from build123d import *

# Parameters (mm, degrees)
ESBO_O1_R                       = 1.75
RESSALTO_EXTRUS_O1_DEPTH        = 8
ESBO_O2_R                       = 1.65
CORTE_EXTRUS_O1_DEPTH           = 7
ESBO_O3_R                       = 1.75
CORTE_EXTRUS_O2_DEPTH           = 18.5
CORTE_EXTRUS_O3_DEPTH           = 2
CORTE_EXTRUS_O3_TAPER           = 20
CORTE_EXTRUS_O3_OTHER_WAY_DEPTH = 6


with BuildPart() as part:
    # Esboço1 → Ressalto-extrusão1 (new body)
    with BuildSketch(Plane.XY):
        with BuildLine():
            Line((17.5, 7.5), (6.986594306, 7.5))
            ThreePointArc((6.986594306, 7.5), (0, 10.25), (-6.986594306, 7.5))
            Line((-6.986594306, 7.5), (-17.5, 7.5))
            Line((-17.5, 7.5), (-17.5, -0.5))
            Line((-17.5, -0.5), (-7.232738071, -0.5))
            ThreePointArc((-7.232738071, -0.5), (-4.946589734, -5.300353762), (0, -7.25))
            Line((0, -7.25), (12.236067977, -7.25))
            Line((12.236067977, -7.25), (12.236067977, -4.75))
            Line((12.236067977, -4.75), (2.236067977, -4.75))
            ThreePointArc((2.236067977, -4.75), (-4.364690104, 2.917529829), (5.244044241, -0.25))
            Line((5.244044241, -0.25), (12.736067977, -0.25))
            Line((12.736067977, -0.25), (12.736067977, -2.25))
            Line((12.736067977, -2.25), (15.807189139, -2.25))
            Line((15.807189139, -2.25), (17.5, -2.25))
            Line((17.5, -2.25), (17.5, 7.5))
        make_face()
        with Locations((12.5, 3.5)):
            Circle(ESBO_O1_R, mode=Mode.SUBTRACT)
        with Locations((-12.5, 3.5)):
            Circle(ESBO_O1_R, mode=Mode.SUBTRACT)
    extrude(amount=RESSALTO_EXTRUS_O1_DEPTH)

    # Esboço2 → Corte-extrusão1 (cut)
    with BuildSketch(Plane(origin=(17.5, 0, 0), x_dir=(0, 0, -1), z_dir=(1, 0, 0))):
        with Locations((-4, 2.625)):
            Circle(ESBO_O2_R)
    corte_extrus_o1 = extrude(amount=-CORTE_EXTRUS_O1_DEPTH, mode=Mode.SUBTRACT)

    # Espelhar1: Corte-extrusão1 across plane
    add(corte_extrus_o1.mirror(Plane(origin=(0, 0, 0), x_dir=(0, 0, 1), z_dir=(1, 0, 0))), mode=Mode.SUBTRACT)

    # Esboço3 → Corte-extrusão2 (cut, through all)
    with BuildSketch(Plane.XZ.offset(7.25)):
        with Locations((7.85, 4)):
            Circle(ESBO_O3_R)
    extrude(amount=-CORTE_EXTRUS_O2_DEPTH, mode=Mode.SUBTRACT)

    # Esboço4 → Corte-extrusão3 (cut)
    with BuildSketch(Plane(origin=(0, 7.5, 0), x_dir=(1, 0, 0), z_dir=(0, 1, 0))):
        Polygon((11.083161507, -4), (9.466580754, -1.2), (6.233419246, -1.2), (4.616838493, -4), (6.233419246, -6.8), (9.466580754, -6.8), align=None)
    extrude(amount=-CORTE_EXTRUS_O3_DEPTH, taper=CORTE_EXTRUS_O3_TAPER, mode=Mode.SUBTRACT)

    # Esboço4 → Corte-extrusão3 other way (cut)
    with BuildSketch(Plane(origin=(0, 7.5, 0), x_dir=(1, 0, 0), z_dir=(0, 1, 0))):
        Polygon((11.083161507, -4), (9.466580754, -1.2), (6.233419246, -1.2), (4.616838493, -4), (6.233419246, -6.8), (9.466580754, -6.8), align=None)
    extrude(amount=CORTE_EXTRUS_O3_OTHER_WAY_DEPTH, mode=Mode.SUBTRACT)


solid = part.part
CAD build for the part. Positions are in the model's coordinates, mm. A direction names the side the tool comes from. Round coordinates to 2 decimals unless told otherwise and drop trailing zeros. Order: outer loops, then holes, each group sorted by start corner. A loop starts at its lowest first (then second) coordinate and runs counter-clockwise, first axis right, second up. Notation, with made-up numbers: (2.25, -4.5) -> (13.25, -4.5) arc R18 ccw to (13.25, 8.5) -> close; hole circle Ø7 at (67, 7.5). An arc over 180 degrees is marked (long way). Write item = value, one per line. Start each with the question number.
(1) Pin check, flat tips, straight feed: P1, Ø1.6, axis at y = 2, z = 3.5, coming from the -X side; P2, Ø1, axis at y = 2.5, z = 4, coming from the +X side; P3, Ø1.2, axis at y = -6.5, z = 4.5, coming from the +X side. Stop position of each tip, or through.
(2) Cut at A-A, the plane x = -12.5. List the corners of the cut face in (y, z) (3 decimals), then the cut area to 3 significant figures.
(3) Probe line 1 (Z direction, x = 7.85, y = 1.4); line 2 (X direction, y = 0.25, z = 6); line 3 (Y direction, x = 8.5, z = 7.75). List the from-to ranges inside material, lowest first. Write a range as [from, to].
(4) Pull direction Z, two halves, no side cores. Call faces 6 (the cylindrical face through (12.272, 5.235, 3.944)), 7 (the flat face through (-10.5, 3, 4)), 8 (the flat face through (0, 6, 0)), 9 (the flat face through (0, 6, 8)): released by +Z, released by -Z, zero draft, split by the parting line, or undercut.
(5) Which spindle directions (+Z, -Z, +X, -X, +Y, -Y) get a long thin tool onto all of the face, cutting with end or side? Do faces 1 (the flat face through (13, 7.5, 4)), 2 (the flat face through (6, -4.75, 3)), 3 (the flat face through (-12, 7.5, 4)), 4 (the flat face through (5.234, 8.131, 5.069)), 5 (the flat face through (10, -0.25, 4)). Say none if no direction does.
(6) Cut at B-B, the plane x = 7.85. State how many separate pieces and enclosed holes the cut face has, then the cut area to 3 significant figures.
Model answer:
q1.P1 = -10.5
q1.P2 = 10.5
q1.P3 = 12.24
q2.outline = (-0.5, 0) -> (1.75, 0) -> (1.75, 2.601) arc R1.65 cw to (1.75, 5.399) -> (1.75, 8) -> (-0.5, 8) -> close; (5.25, 0) -> (7.5, 0) -> (7.5, 8) -> (5.25, 8) -> close
q2.area = 34.5 mm2
q3.line_1 = [0, 2.25], [5.75, 8]
q3.line_2 = [-17.5, -5.24], [5.24, 17.5]
q3.line_3 = [-7.25, -4.75], [-0.25, 7.5]
q4.face_6 = zero draft
q4.face_7 = undercut
q4.face_8 = released by -Z
q4.face_9 = released by +Z
q5.face_1 = +Z, -Z, +X, +Y
q5.face_2 = +Z, -Z, +X
q5.face_3 = +Z, -Z, -X, +Y
q5.face_4 = +X, +Y
q5.face_5 = +Z, -Z
q6.separate_pieces = 4
q6.enclosed_holes = 0
q6.area = 43.4 mm2
